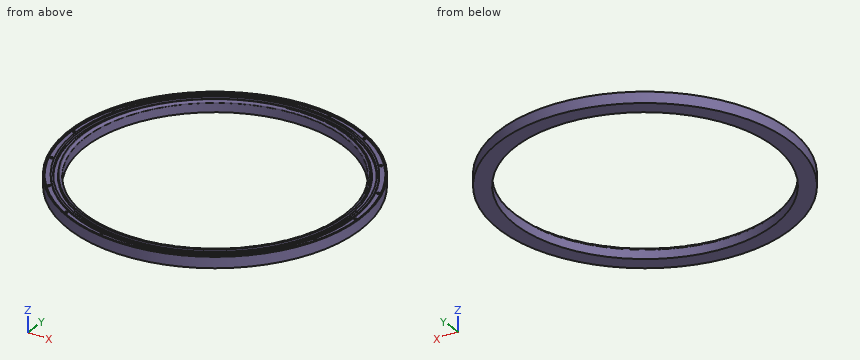
```python
from build123d import *

# Parameters (mm, degrees)
F0_R     = 225
F0_R_2   = 200
F1_DEPTH = 17
F2_R     = 211.9
F2_R_2   = 205
F3_DEPTH = 4
F4_R     = 0.6
F5_R     = 223
F5_R_2   = 215
F6_DEPTH = 2
F7_R     = 3
F9_D     = 4.2
F9_DEPTH = 8.6
F9_TIP   = 1.2618073


# Not quite as in the source:
# - a feature names something its author has since deleted; it is built from what else it names


with BuildPart() as f1:
    # F0 (on Top) → F1 (new body)
    with BuildSketch(Plane.XY):
        Circle(F0_R)
        Circle(F0_R_2, mode=Mode.SUBTRACT)
    extrude(amount=F1_DEPTH)

    # F2 (on face) → F3 (cut)
    with BuildSketch(Plane.XY.offset(17)):
        Circle(F2_R)
        Circle(F2_R_2, mode=Mode.SUBTRACT)
    extrude(amount=-F3_DEPTH, mode=Mode.SUBTRACT)

    # F4
    f4_edges = [f1.edges().sort_by_distance(p)[0] for p in [
        (-211.9, 0, 13),
        (-205, 0, 13),
    ]]
    fillet(f4_edges, radius=F4_R)

    # F5 (on face) → F6 (cut)
    with BuildSketch(Plane.XY.offset(17)):
        Circle(F5_R)
        Circle(F5_R_2, mode=Mode.SUBTRACT)
    extrude(amount=-F6_DEPTH, mode=Mode.SUBTRACT)

    # F7
    f7_edges = [f1.edges().sort_by_distance(p)[0] for p in [
        (-200, 0, 17),
    ]]
    fillet(f7_edges, radius=F7_R)

    # F9
    with Locations(Plane.XY.offset(15)):
        with Locations((219, 0), (205.7926839521, 74.9024113883), (167.7637330431, 140.7704865214), (109.5, 189.6595634288), (38.0289509091, 215.6728979097), (-38.0289509091, 215.6728979097), (-109.5, 189.6595634288), (-167.7637330431, 140.7704865214), (-205.7926839521, 74.9024113883), (-219, 0), (-205.7926839521, -74.9024113883), (-167.7637330431, -140.7704865214), (-109.5, -189.6595634288), (-38.0289509091, -215.6728979097), (38.0289509091, -215.6728979097), (109.5, -189.6595634288), (167.7637330431, -140.7704865214), (205.7926839521, -74.9024113883)):
            Hole(F9_D / 2, depth=F9_DEPTH)
            with Locations((0, 0, -(F9_DEPTH + F9_TIP / 2))):  # 118° drill point
                Cone(0, F9_D / 2, F9_TIP, mode=Mode.SUBTRACT)


solid = f1.part
```
The listing builds one solid part. Answer for the finished solid, in the listing's coordinates (mm). Give positions to 0.01 mm unless a question says otherwise; leave off trailing zeros. Answer in a Markdown table with one row per item. Add a question column.
Q1. Given P1, Ø5.5, axis at x = 167.76, y = -140.77, coming from the +Z side; P2, Ø1, axis at y = 72, z = 4.5, coming from the +X side; P3, Ø2.5, axis at x = 205.79, y = -74.9, coming from the +Z side, each flat-ended and moving along its own axis, determine where each tip first touches the part or whether it passes through.
Q2. Find the intervals of material crossed by line 1 along Y through (x, z) = (113, 14); line 2 along X through (y, z) = (96, 16.25); line 3 along Y through (x, z) = (-145.5, 13.5), in increasing order. Write a range as [from, to].
Q3. The part is cut by section B-B (z = 9). Give the number of separate pieces and of enclosed holes in the cut face, then the cut area to 3 significant figures.
Determined:
| question | item | result |
|---|---|---|
| 1 | P1 | stops at z = 15 |
| 1 | P2 | stops at x = 213.34 |
| 1 | P3 | stops at z = 5.89 |
| 2 | line 1 | y = [-194.57, -179.26], [-171.04, -165.02], [165.02, 171.04], [179.26, 194.57] |
| 2 | line 2 | x = [-203.49, -201.28], [-192.38, -188.91], [-181.13, -176.61], [176.61, 181.13], [188.91, 192.38], [201.28, 203.49] |
| 2 | line 3 | y = [-171.62, -154.04], [-144.42, -137.22], [137.22, 144.42], [154.04, 171.62] |
| 3 | separate pieces | 1 |
| 3 | enclosed holes | 19 |
| 3 | area | 33,100 mm² |
